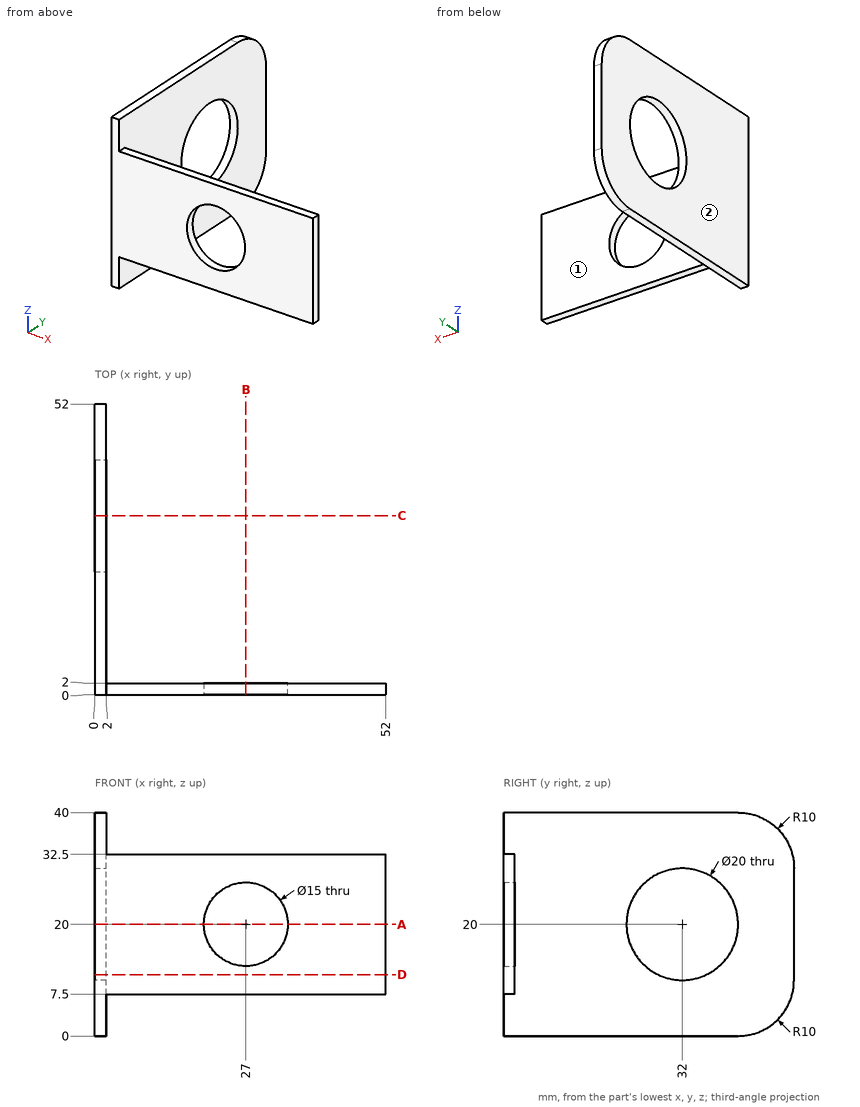
Print and shaded views of the part. All mm, measured from the part's lowest x, y and z. A direction names the side the tool comes from. Round coordinates to 2 decimals unless told otherwise and drop trailing zeros. Write each loop counter-clockwise with the first axis right and the second up, starting at its lowest first coordinate (ties: lowest second). Pieces come first, ordered by that corner, then holes. Notation, with made-up numbers: M -1.75,58.25 L 13.25,58.25 A20 cw 13.25,97.25 Z; hole C -27.5,47 d7. An arc over 180 degrees is marked long. Use a Markdown table: item, result. Add a question column.
1. Slice it at D-D on z = 11. Give the cut face in (x, y).
2. Slice it at A-A on z = 20. Give the cut face in (x, y).
3. Drill centre lines: probe 1 along Y at (x, z) = (0.8, 20); probe 2 along Y at (x, z) = (34, 28). Where is each one in solid material? Low to high.
4. Slice it at B-B on x = 27. Give the cut face in (y, z), then the cut area to 3 significant figures.
5. Slice it at C-C on y = 32. Give the cut face in (x, z), then the cut area to 3 significant figures.
6. 3-axis set-ups, long thin cutter, end or side, ignore diameter. For the marked faces 1 and 2: which of +Z, -Z, +X, -X, +Y, -Y reach the whole face in a straight line?
7. Flat gauge pins, fed straight in: P1, Ø1, axis at x = 25.5, y = 1, coming from the -Z side; P2, Ø10, axis at y = 31.5, z = 30.5, coming from the +X side; P3, Ø6, axis at y = 32, z = 14.5, coming from the +X side; P4, Ø10, axis at x = 10, z = 7.5, coming from the +Y side. Where does each tip first touch, or does it go through?
Reply:
| question | item | result |
|---|---|---|
| 1 | outline | M 0,0 L 52,0 L 52,2 L 2,2 L 2,27.64 L 0,27.64 Z; M 0,36.36 L 2,36.36 L 2,52 L 0,52 Z |
| 2 | outline | M 0,0 L 19.5,0 L 19.5,2 L 2,2 L 2,22 L 0,22 Z; M 0,42 L 2,42 L 2,52 L 0,52 Z; M 34.5,0 L 52,0 L 52,2 L 34.5,2 Z |
| 3 | probe 1 | y = 0 to 22, 42 to 52 |
| 3 | probe 2 | y = 0 to 2 |
| 4 | outline | M 0,7.5 L 2,7.5 L 2,12.5 L 0,12.5 Z; M 0,27.5 L 2,27.5 L 2,32.5 L 0,32.5 Z |
| 4 | area | 20.0 mm^2 |
| 5 | outline | M 0,0 L 2,0 L 2,10 L 0,10 Z; M 0,30 L 2,30 L 2,40 L 0,40 Z |
| 5 | area | 40.0 mm^2 |
| 6 | face 1 | +Z, -Z, +X, +Y |
| 6 | face 2 | +Z, -Z, -X, +Y, -Y |
| 7 | P1 | stops at z = 7.5 |
| 7 | P2 | stops at x = 2 |
| 7 | P3 | passes through |
| 7 | P4 | stops at y = 2 |
